Could you check a few things on this model? Use its own coordinates, in mm. Face numbers are marked on the shaded views. A direction names the side the tool comes from. Round coordinates to 2 decimals unless told otherwise and drop trailing zeros. Write each loop counter-clockwise with the first axis right and the second up, starting at its lowest first coordinate (ties: lowest second). Pieces come first, ordered by that corner, then holes. Notation, with made-up numbers: (52, 59) -> (108, 59) arc R20 cw to (108, 77) -> close; hole circle Ø6 at (68, 67). An arc over 180 degrees is marked (long way). Answer in a Markdown table with one row per item.
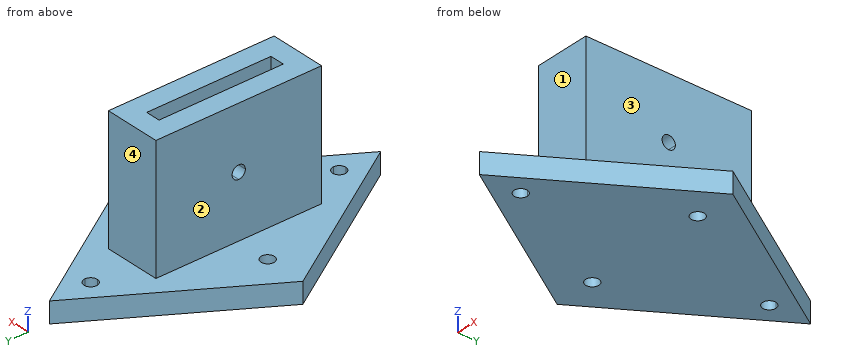
from build123d import *

# Parameters (mm, degrees)
F1_DEPTH = 5
F3_DEPTH = 30
F5_DEPTH = 31.751


with BuildPart() as f1:
    # F0 (on Top) → F1 (new body)
    with BuildSketch(Plane.XY):
        with BuildLine():
            ThreePointArc((-16.6, 0), (-15, 1.6), (-13.4, 0))
            Line((-13.4, 0), (0, 0))
            Line((0, 0), (0, 28.4))
            ThreePointArc((0, 28.4), (-1.6, 30), (0, 31.6))
            Line((0, 31.6), (0, 40))
            Line((0, 40), (-25, 0))
            Line((-25, 0), (-16.6, 0))
        make_face()
        with BuildLine():
            Line((0, 0), (-13.4, 0))
            ThreePointArc((-13.4, 0), (-15, -1.6), (-16.6, 0))
            Line((-16.6, 0), (-25, 0))
            Line((-25, 0), (0, -40))
            Line((0, -40), (0, -31.6))
            ThreePointArc((0, -31.6), (-1.6, -30), (0, -28.4))
            Line((0, -28.4), (0, 0))
        make_face()
        with BuildLine():
            Line((0, 28.4), (0, 0))
            Line((0, 0), (13.4, 0))
            ThreePointArc((13.4, 0), (15, 1.6), (16.6, 0))
            Line((16.6, 0), (25, 0))
            Line((25, 0), (0, 40))
            Line((0, 40), (0, 31.6))
            ThreePointArc((0, 31.6), (1.131371, 31.131371), (1.6, 30))
            ThreePointArc((1.6, 30), (1.131371, 28.868629), (0, 28.4))
        make_face()
        with BuildLine():
            Line((13.4, 0), (0, 0))
            Line((0, 0), (0, -28.4))
            ThreePointArc((0, -28.4), (1.131371, -28.868629), (1.6, -30))
            ThreePointArc((1.6, -30), (1.131371, -31.131371), (0, -31.6))
            Line((0, -31.6), (0, -40))
            Line((0, -40), (25, 0))
            Line((25, 0), (16.6, 0))
            ThreePointArc((16.6, 0), (15, -1.6), (13.4, 0))
        make_face()
    extrude(amount=F1_DEPTH)

    # F2 (on face) → F3 (join)
    with BuildSketch(Plane.XY.offset(5)):
        Polygon((6.75, 20), (0, 20), (0, 15), (1.75, 15), (1.75, 0), (6.75, 0), align=None)
        Polygon((0, 15), (0, 20), (-6.75, 20), (-6.75, 0), (-1.75, 0), (-1.75, 15), align=None)
        Polygon((6.75, -20), (6.75, 0), (1.75, 0), (1.75, -15), (0, -15), (0, -20), align=None)
        Polygon((-1.75, 0), (-6.75, 0), (-6.75, -20), (0, -20), (0, -15), (-1.75, -15), align=None)
    extrude(amount=F3_DEPTH)

    # F4 (on face) → F5 (cut, through all)
    with BuildSketch(Plane(origin=(-6.75, 0, 0), x_dir=(0, -1, 0), z_dir=(-1, 0, 0))):
        with BuildLine():
            ThreePointArc((-1.6, 20), (-1.131371, 18.868629), (0, 18.4))
            Line((0, 18.4), (0, 20))
            Line((0, 20), (-1.6, 20))
        make_face()
        with BuildLine():
            Line((0, 20), (0, 18.4))
            ThreePointArc((0, 18.4), (1.131371, 18.868629), (1.6, 20))
            ThreePointArc((1.6, 20), (0, 21.6), (-1.6, 20))
            Line((-1.6, 20), (0, 20))
        make_face()
    extrude(amount=-F5_DEPTH, mode=Mode.SUBTRACT)


solid = f1.part
1) Imagine slicing it at B-B, the plane z = 3. Please give me the cut outline in (x, y), plus the area to 3 significant figures.
Findings:
| item | result |
|---|---|
| outline | (-25, 0) -> (0, -40) -> (25, 0) -> (0, 40) -> close; hole circle Ø3.2 at (-15, 0); hole (0, -28.4) arc R1.6 ccw (long way) to (1.6, -30) arc R1.6 ccw to start; hole (0, 31.6) arc R1.6 ccw (long way) to (1.6, 30) arc R1.6 ccw to start; hole circle Ø3.2 at (15, 0) |
| area | 1,970 mm^2 |
2) Imagine slicing it at A-A, the plane x = -15. Please give me the cut outline in (y, z), plus the area to 3 significant figures.
Findings:
| item | result |
|---|---|
| outline | (-16, 0) -> (-1.6, 0) -> (-1.6, 5) -> (-16, 5) -> close; (1.6, 0) -> (16, 0) -> (16, 5) -> (1.6, 5) -> close |
| area | 144 mm^2 |
3) For pin 1 (11 mm diameter, centred on x = -0.5, z = 15.5, fed in from -Y); pin 2 (9 mm diameter, centred on y = 8, z = 19, fed in from +X); pin 3 (1 mm diameter, centred on x = -1, y = 1.5, fed in from +Z), each with a flat end and sliding along its axis, tell me the tip position at first contact or that it passes through.
Findings:
| item | result |
|---|---|
| pin 1 | stops at y = -20 |
| pin 2 | stops at x = 6.75 |
| pin 3 | stops at z = 5 |
4) Imagine slicing it at C-C, the plane x = 4. Please give me the cut outline in (y, z), plus the area to 3 significant figures.
Findings:
| item | result |
|---|---|
| outline | (-33.6, 0) -> (33.6, 0) -> (33.6, 5) -> (20, 5) -> (20, 35) -> (-20, 35) -> (-20, 5) -> (-33.6, 5) -> close; hole (0, 18.4) arc R1.6 ccw to (1.6, 20) arc R1.6 ccw (long way) to start |
| area | 1,530 mm^2 |
5) Please list where these lines run through material, in increasing order: line 1 (X direction, y = 3.5, z = 26.5); line 2 (Z direction, x = 3, y = 0); line 3 (Y direction, x = 1, z = 16).
Findings:
| item | result |
|---|---|
| line 1 | x = -6.75 to -1.75, 1.75 to 6.75 |
| line 2 | z = 0 to 18.4, 21.6 to 35 |
| line 3 | y = -20 to -15, 15 to 20 |
6) Imagine slicing it at D-D, the plane y = 14. Please give me the cut outline in (x, z), plus the area to 4 significant figures.
Findings:
| item | result |
|---|---|
| outline | (-16.25, 0) -> (16.25, 0) -> (16.25, 5) -> (6.75, 5) -> (6.75, 35) -> (1.75, 35) -> (1.75, 5) -> (-1.75, 5) -> (-1.75, 35) -> (-6.75, 35) -> (-6.75, 5) -> (-16.25, 5) -> close |
| area | 462.5 mm^2 |
7) For the marked faces 1, 2, 3 and 4, which set-ups out of +Z, -Z, +X, -X, +Y, -Y let a thin tool reach every point of the face, with its end or its side?
Findings:
| item | result |
|---|---|
| face 1 | +Z, +X, -X, -Y |
| face 2 | +Z, -X, +Y, -Y |
| face 3 | +Z, +X, +Y, -Y |
| face 4 | +Z, +X, -X, +Y |
